from build123d import *

# Parameters (mm, degrees)
SKETCH_1_R          = 20
EXTRUDE_1_DEPTH     = 45
SKETCH_3_R          = 35
EXTRUDE_2_DEPTH     = 44
SKETCH_4_R          = 19
EXTRUDE_3_DEPTH     = 91
SKETCH_5_R          = 4
CUT_EXTRUDE_1_DEPTH = 91
SKETCH_6_R          = 10
CUT_EXTRUDE_2_DEPTH = 180
CUT_EXTRUDE_3_DEPTH = 30
CHAMFER_1_SIZE      = 1
SKETCH_8_W          = 12
SKETCH_8_H          = 40
CUT_EXTRUDE_4_DEPTH = 5


with BuildPart() as part:
    # Эскиз1 → Бобышка-Вытянуть1 (new body)
    with BuildSketch(Plane.XY):
        Circle(SKETCH_1_R)
    extrude(amount=-EXTRUDE_1_DEPTH)

    # Эскиз3 → Бобышка-Вытянуть2 (add)
    with BuildSketch(Plane(origin=(0, 0, -45), x_dir=(-1, 0, 0), z_dir=(0, 0, -1))):
        Circle(SKETCH_3_R)
    extrude(amount=EXTRUDE_2_DEPTH)

    # Эскиз4 → Бобышка-Вытянуть3 (add)
    with BuildSketch(Plane(origin=(0, 0, -89), x_dir=(-1, 0, 0), z_dir=(0, 0, -1))):
        Circle(SKETCH_4_R)
    extrude(amount=EXTRUDE_3_DEPTH)

    # Эскиз5 → Вырез-Вытянуть1 (cut)
    with BuildSketch(Plane(origin=(0, 35, 0), x_dir=(1, 0, 0), z_dir=(0, 1, 0))):
        with Locations((0, 67)):
            Circle(SKETCH_5_R)
    extrude(amount=-CUT_EXTRUDE_1_DEPTH, mode=Mode.SUBTRACT)

    # Эскиз6 → Вырез-Вытянуть2 (cut)
    with BuildSketch(Plane(origin=(0, 0, -180), x_dir=(-1, 0, 0), z_dir=(0, 0, -1))):
        Circle(SKETCH_6_R)
    extrude(amount=-CUT_EXTRUDE_2_DEPTH, mode=Mode.SUBTRACT)

    # Эскиз7 → Вырез-Вытянуть3 (cut)
    with BuildSketch(Plane.XY):
        with BuildLine():
            Line((-15, 13.228756555), (-15, -13.228756555))
            ThreePointArc((-15, -13.228756555), (-20, 0), (-15, 13.228756555))
        make_face()
        with BuildLine():
            Line((15, 13.228756555), (15, -13.228756555))
            ThreePointArc((15, -13.228756555), (20, 0), (15, 13.228756555))
        make_face()
    extrude(amount=-CUT_EXTRUDE_3_DEPTH, mode=Mode.SUBTRACT)

    # Фаска1
    chamfer_1_edges = [part.edges().sort_by_distance(p)[0] for p in [
        (19, 0, -180),
        (0, 20, 0),
        (0, -20, 0),
    ]]
    chamfer(chamfer_1_edges, length=CHAMFER_1_SIZE)

    # Эскиз8 → Вырез-Вытянуть4 (cut)
    with BuildSketch(Plane(origin=(0, 19, 0), x_dir=(1, 0, 0), z_dir=(0, 1, 0))):
        with Locations((0, 145)):
            Rectangle(SKETCH_8_W, SKETCH_8_H)
    extrude(amount=-CUT_EXTRUDE_4_DEPTH, mode=Mode.SUBTRACT)


solid = part.part
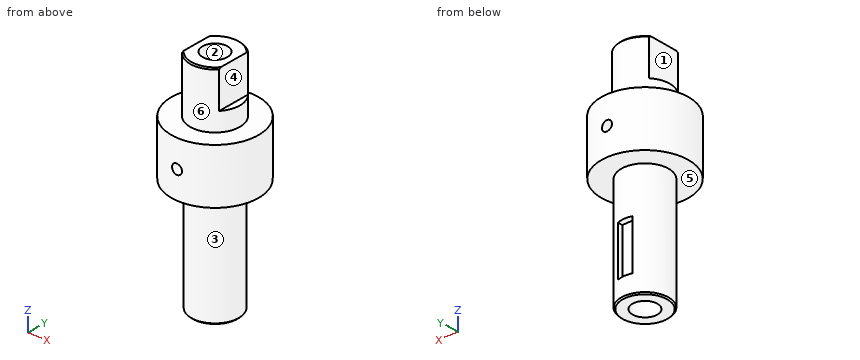
Check sheet for the modelled part. Datum: model origin and axes. Units: mm. Face numbers are marked on the shaded views. A direction names the side the tool comes from. Give positions to 0.01 mm unless a question says otherwise; leave off trailing zeros. Loops run counter-clockwise (first coordinate to the right, second up) from the corner with the lowest first, then second, coordinate; pieces in that order, holes last. Notation, with made-up numbers: M 56.5,-19 L 96.5,-19 A23 ccw 96.5,3 Z; hole C 32,22.25 d4. An arc over 180 degrees is marked long. Answer as a JSON object with one key per item and string values. Group by question number.
Q1. Access from +Z, -Z, +X, -X, +Y, -Y to the whole of each face (thin tool, end or side, straight path). Record for the marked faces 4, 5 and 6.
Q2. Cross-section at A-A on y = 0. Record the cut outline in (x, z), then the cut area to 3 significant figures.
Q3. Cross-section at C-C on z = -67. Record the cut outline in (x, y).
Q4. Cross-section at D-D on z = -153. Record the cut outline in (x, y).
Q5. Cross-section at B-B on x = 0. Give the number of separate pieces and of enclosed holes in the cut face, then the cut area to 3 significant figures.
Q6. Release check for a two-part mould opening along Y. For the marked faces 1, 2 and 3 record: released by +Y, released by -Y, zero draft, split by the parting line, or undercut.
Q7. Material ranges on line 1 along Z through (x, y) = (0, 17.5); line 2 along Z through (x, y) = (0, 26); line 3 along Y through (x, z) = (0, -53.5), recorded low to high. Write a range as [from, to].
Q8. Go/stop test with flat-tipped pins: P1, Ø4, axis at y = 13, z = -44, coming from the +X side; P2, Ø5, axis at x = 0, z = -67, coming from the +Y side; P3, Ø13, axis at y = 1.5, z = -22, coming from the -X side; P4, Ø8, axis at y = 4, z = -125.5, coming from the +X side. Record where each tip stops, or that it passes through.
Evaluation:
{
 "1": {"face 4": "+Z, +X, +Y, -Y", "face 5": "-Z", "face 6": "+Z"},
 "2": {"outline": "M -35,-89 L -19,-89 L -19,-179 L -18,-180 L -10,-180 L -10,0 L -15,0 L -15,-30 L -20,-30 L -20,-45 L -35,-45 Z; M 10,-180 L 18,-180 L 19,-179 L 19,-89 L 35,-89 L 35,-45 L 20,-45 L 20,-30 L 15,-30 L 15,0 L 10,0 Z", "area": "4,440 mm2"},
 "3": {"outline": "M -4,-34.77 L -4,-9.17 A10 cw -4,9.17 L -4,34.77 A35 ccw Z; M 4,-34.77 A35 ccw 4,34.77 L 4,9.17 A10 cw 4,-9.17 Z"},
 "4": {"outline": "M -6,14 L -6,18.03 A19 ccw long 6,18.03 L 6,14 Z; hole C 0,0 d20"},
 "5": {"separate pieces": "4", "enclosed holes": "0", "area": "4,140 mm2"},
 "6": {"face 1": "zero draft", "face 2": "undercut", "face 3": "split by the parting line"},
 "7": {"line 1": "z = [-180, -165], [-125, -71], [-63, 0]", "line 2": "z = [-89, -71], [-63, -45]", "line 3": "y = [-35, -10], [10, 35]"},
 "8": {"P1": "stops at x = 33.14", "P2": "passes through", "P3": "stops at x = -15", "P4": "stops at x = 19"}
}
